Study the drawing (mm; zero at the part's minimum x, y, z) and answer. Give positions to 0.01 mm unless a question says otherwise; leave off trailing zeros. Order: outer loops, then holes, each group sorted by start corner. A loop starts at its lowest first (then second) coordinate and runs counter-clockwise, first axis right, second up. Notation, with made-up numbers: (61.5, -26) - (114.5, -26) arc R22 ccw to (114.5, 6) - close; hole circle Ø2 at (77.5, 37). An arc over 180 degrees is marked (long way). Return JSON: item names as keys, results as strings.
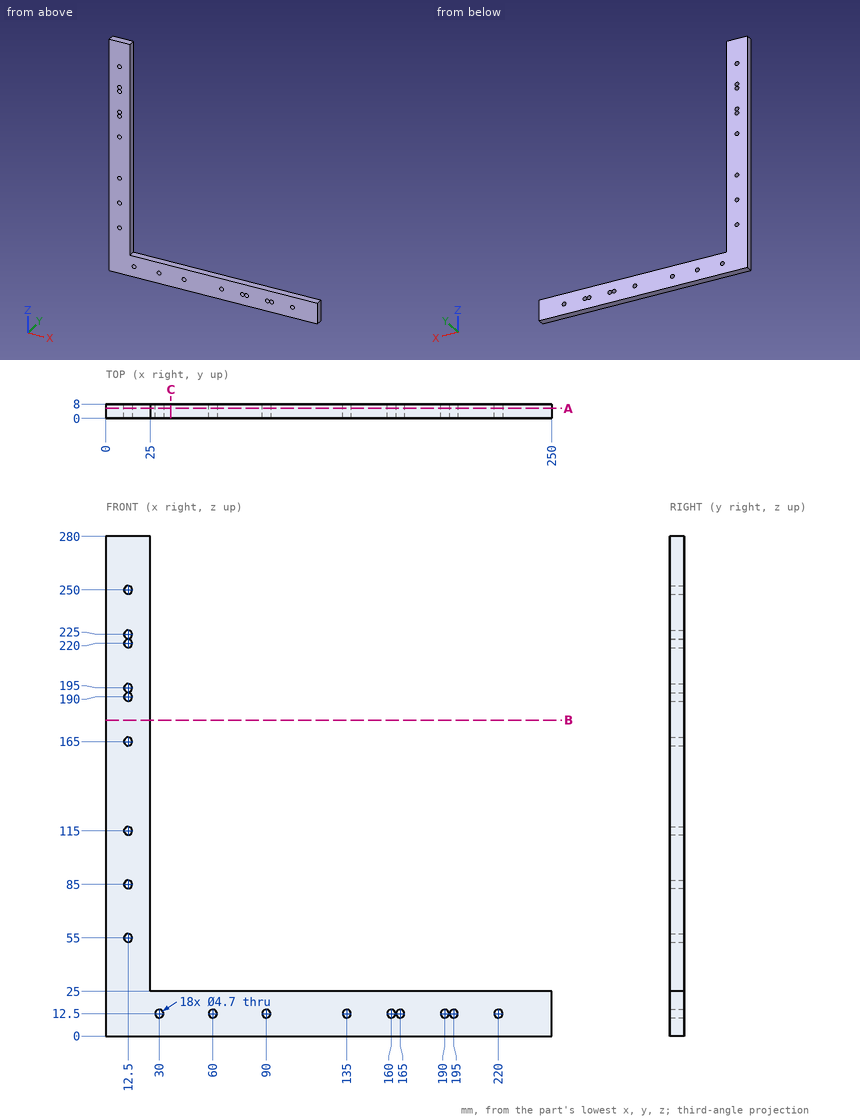
Q1. A cutting plane is placed at A-A (y = 5.5). Give the number of separate pieces and of enclosed holes in the cut face, and give its area (3 significant figures).
Values:
{"separate pieces": "1", "enclosed holes": "18", "area": "12,300 mm²"}
Q2. Consider L1, parallel to Z at x = 165, y = 2.75; L2, parallel to Z at x = 110, y = 0.75. Determine where each line is inside the solid, lowest interval first.
Values:
{"L1": "z = 0 to 10.15, 14.85 to 25", "L2": "z = 0 to 25"}
Q3. A cutting plane is placed at B-B (z = 177). Write down the section's boundary in (x, y).
Values:
{"outline": "(0, 0) - (25, 0) - (25, 8) - (0, 8) - close"}
Q4. Given pin 1 (1.5 mm diameter, centred on y = 4.5, z = 78, fed in from +X); pin 2 (2 mm diameter, centred on x = 72.5, y = 3, fed in from +Z), each flat-ended and moving along its own axis, determine where each tip first touches the part or whether it passes through.
Values:
{"pin 1": "stops at x = 25", "pin 2": "stops at z = 25"}
Q5. A cutting plane is placed at C-C (x = 36.5). Write down the section's boundary in (y, z).
Values:
{"outline": "(0, 0) - (8, 0) - (8, 25) - (0, 25) - close"}
